from build123d import *

# Parameters (mm, degrees)
EXTRUDE_1_DEPTH     = 2
SKETCH_2_W          = 46
SKETCH_2_H          = 21
EXTRUDE_2_DEPTH     = 5.5
SKETCH_3_R          = 2.5
SKETCH_3_R_2        = 1.5
EXTRUDE_3_DEPTH     = 5.5
CUT_EXTRUDE_2_REACH = 27
SKETCH_5_W          = 12.7
SKETCH_5_H          = 3
EXTRUDE_4_DEPTH     = 7.5
SKETCH_7_R          = 1.5
CUT_EXTRUDE_3_DEPTH = 3
EXTRUDE_5_DEPTH     = 18
EXTRUDE_6_DEPTH     = 18
SKETCH_10_W         = 5
SKETCH_10_H         = 7.5
SKETCH_10_R         = 1.5
EXTRUDE_7_DEPTH     = 5


with BuildPart() as part:
    # 草图1 → 凸台-拉伸1 (new body)
    with BuildSketch(Plane(origin=(0, 0, 0), x_dir=(1, 0, 0), z_dir=(0, 1, 0))):
        with BuildLine():
            Line((-23, 12.5), (23, 12.5))
            ThreePointArc((23, 12.5), (24.414213562, 11.914213562), (25, 10.5))
            Line((25, 10.5), (25, -10.5))
            ThreePointArc((25, -10.5), (24.414213562, -11.914213562), (23, -12.5))
            Line((23, -12.5), (-23, -12.5))
            ThreePointArc((-23, -12.5), (-24.414213562, -11.914213562), (-25, -10.5))
            Line((-25, -10.5), (-25, 10.5))
            ThreePointArc((-25, 10.5), (-24.414213562, 11.914213562), (-23, 12.5))
        make_face()
    extrude(amount=EXTRUDE_1_DEPTH)

    # 草图2 → 凸台-拉伸2 (add)
    with BuildSketch(Plane(origin=(0, 2, 0), x_dir=(1, 0, 0), z_dir=(0, 1, 0))):
        with BuildLine():
            Line((-25, 10.5), (-25, -10.5))
            ThreePointArc((-25, -10.5), (-24.414213562, -11.914213562), (-23, -12.5))
            Line((-23, -12.5), (23, -12.5))
            ThreePointArc((23, -12.5), (24.414213562, -11.914213562), (25, -10.5))
            Line((25, -10.5), (25, 10.5))
            ThreePointArc((25, 10.5), (24.414213562, 11.914213562), (23, 12.5))
            Line((23, 12.5), (-23, 12.5))
            ThreePointArc((-23, 12.5), (-24.414213562, 11.914213562), (-25, 10.5))
        make_face()
        Rectangle(SKETCH_2_W, SKETCH_2_H, mode=Mode.SUBTRACT)
    extrude(amount=EXTRUDE_2_DEPTH)

    # 草图3 → 凸台-拉伸3 (add)
    with BuildSketch(Plane(origin=(0, 2, 0), x_dir=(1, 0, 0), z_dir=(0, 1, 0))):
        with Locations((-21, 8.5)):
            Circle(SKETCH_3_R)
        with Locations((-21, 8.5)):
            Circle(SKETCH_3_R_2, mode=Mode.SUBTRACT)
        with Locations((21, 8.5)):
            Circle(SKETCH_3_R)
        with Locations((21, 8.5)):
            Circle(SKETCH_3_R_2, mode=Mode.SUBTRACT)
        with Locations((21, -8.5)):
            Circle(SKETCH_3_R)
        with Locations((21, -8.5)):
            Circle(SKETCH_3_R_2, mode=Mode.SUBTRACT)
        with Locations((-21, -8.5)):
            Circle(SKETCH_3_R)
        with Locations((-21, -8.5)):
            Circle(SKETCH_3_R_2, mode=Mode.SUBTRACT)
    extrude(amount=EXTRUDE_3_DEPTH)

    # 草图5 → 切除-拉伸2 (cut, up to next)
    with BuildSketch(Plane.XY.offset(12.5), mode=Mode.PRIVATE) as cut_extrude_2_sk1:
        with Locations((0, 3.5)):
            Rectangle(SKETCH_5_W, SKETCH_5_H)
    cut_extrude_2_tool1 = extrude(cut_extrude_2_sk1.sketch, amount=-CUT_EXTRUDE_2_REACH, mode=Mode.PRIVATE) & part.part
    add(cut_extrude_2_tool1.solids().sort_by_distance((0, 3.5, 12.5))[0], mode=Mode.SUBTRACT)

    # 草图6 → 凸台-拉伸4 (add)
    with BuildSketch(Plane.XZ):
        Polygon((23, 12.5), (30, 12.5), (30, 10.5), (25, 10.5), align=None)
        Polygon((-23, 12.5), (-30, 12.5), (-30, 10.5), (-25, 10.5), align=None)
    extrude(amount=-EXTRUDE_4_DEPTH)

    # 草图7 → 切除-拉伸3 (cut, through all)
    with BuildSketch(Plane(origin=(0, 0, 10.5), x_dir=(-1, 0, 0), z_dir=(0, 0, -1))):
        with Locations((-27.5, 3.75)):
            Circle(SKETCH_7_R)
        with Locations((27.5, 3.75)):
            Circle(SKETCH_7_R)
    extrude(amount=-CUT_EXTRUDE_3_DEPTH, mode=Mode.SUBTRACT)

    # 草图8 → 凸台-拉伸5 (add)
    with BuildSketch(Plane.XY.offset(12.5)):
        with BuildLine():
            Line((-29, 7.5), (-29, 3.75))
            ThreePointArc((-29, 3.75), (-27.5, 2.25), (-26, 3.75))
            Line((-26, 3.75), (-26, 7.5))
            Line((-26, 7.5), (-24, 7.5))
            Line((-24, 7.5), (-24, 0))
            Line((-24, 0), (-30, 0))
            Line((-30, 0), (-30, 7.5))
            Line((-30, 7.5), (-29, 7.5))
        make_face()
        with BuildLine():
            Line((29, 7.5), (29, 3.75))
            ThreePointArc((29, 3.75), (27.5, 2.25), (26, 3.75))
            Line((26, 3.75), (26, 7.5))
            Line((26, 7.5), (24, 7.5))
            Line((24, 7.5), (24, 0))
            Line((24, 0), (30, 0))
            Line((30, 0), (30, 7.5))
            Line((30, 7.5), (29, 7.5))
        make_face()
    extrude(amount=EXTRUDE_5_DEPTH)

    # 草图9 → 凸台-拉伸6 (add)
    with BuildSketch(Plane.XY.offset(12.5)):
        with BuildLine():
            Line((29, 3.75), (29, 7.5))
            Line((29, 7.5), (26, 7.5))
            Line((26, 7.5), (26, 3.75))
            ThreePointArc((26, 3.75), (27.5, 5.25), (29, 3.75))
        make_face()
        with BuildLine():
            Line((-29, 7.5), (-29, 3.75))
            ThreePointArc((-29, 3.75), (-27.5, 5.25), (-26, 3.75))
            Line((-26, 3.75), (-26, 7.5))
            Line((-26, 7.5), (-29, 7.5))
        make_face()
    extrude(amount=EXTRUDE_6_DEPTH)

    # 草图10 → 凸台-拉伸7 (add)
    with BuildSketch(Plane(origin=(0, 0, 10.5), x_dir=(-1, 0, 0), z_dir=(0, 0, -1))):
        with Locations((-27.5, 3.75)):
            Rectangle(SKETCH_10_W, SKETCH_10_H)
        with Locations((-27.5, 3.75)):
            Circle(SKETCH_10_R, mode=Mode.SUBTRACT)
        with Locations((27.5, 3.75)):
            Rectangle(SKETCH_10_W, SKETCH_10_H)
        with Locations((27.5, 3.75)):
            Circle(SKETCH_10_R, mode=Mode.SUBTRACT)
    extrude(amount=EXTRUDE_7_DEPTH)


solid = part.part
Input: part model. Units: mm. Frame: model coordinates. A direction names the side the tool comes from. Coordinates: 2 decimals unless noted, no trailing zeros. Loops run counter-clockwise (first coordinate to the right, second up) from the corner with the lowest first, then second, coordinate; pieces in that order, holes last. Notation, with made-up numbers: (-21.75, 53) - (-13.75, 53) arc R23 cw to (-13.75, 66) - close; hole circle Ø11 at (-37, 33.5). An arc over 180 degrees is marked (long way). Answer in a Markdown table with one row per item. Add a question column.
Item 1: Contact query for flat-ended pins moving along their axis: P1, Ø0.9, axis at x = 21, z = 9, coming from the +Y side; P2, Ø3, axis at y = 3.5, z = 0.5, coming from the +X side; P3, Ø1, axis at x = 11.5, y = 4.5, coming from the +Z side. Output: stop coordinate, or through.
Item 2: Section query D-D on z = 8.5. Return the cut outline in (x, y).
Item 3: Section query A-A on x = -27.5. Return the cut outline in (y, z).
Item 4: Access query for faces 5 (the cylindrical face through (-22.5, 4.71, 8.43)), 6 (the flat face through (28, 2, 5.5)), 7 (the flat face through (0, 5, 12)), 8 (the flat face through (-24, 4, 21)). Directions: +Z, -Z, +X, -X, +Y, -Y. A direction counts if a zero-diameter tool reaches every point of the face in a straight line with its end or side. Return the directions, or none.
Item 5: Section query C-C on z = -1.5. Return the cut outline in (x, y).
Item 6: Line query: line 1 along X through (y, z) = (5, -8.5); line 2 along X through (y, z) = (6.3, 8.5); line 3 along Z through (x, y) = (-21, 5.9). Output: solid intervals per line, ascending. Write a range as [from, to].
Item 7: Section query B-B on y = 3.75. State how many separate pieces and enclosed holes the cut face has, then the cut area to 3 significant figures.
Item 8: Mould query, pull axis X, two halves, no side actions, for faces 1 (the flat face through (25.6, 3.8, 30.5)), 2 (the flat face through (-21, 2, 8)), 3 (the cylindrical face through (-22.5, 4.71, -8.57)), 4 (the flat face through (-25, 4, -3)). Classes: released by +X, released by -X, zero draft, split by the parting line, or undercut.
Recorded:
| question | item | result |
|---|---|---|
| 1 | P1 | y = 2 |
| 1 | P2 | x = 25 |
| 1 | P3 | z = 12.5 |
| 2 | outline | (-30, 0) - (30, 0) - (30, 7.5) - (22.5, 7.5) - (22.5, 2) - (19.5, 2) - (19.5, 7.5) - (18.5, 7.5) - (18.5, 2) - (-18.5, 2) - (-18.5, 7.5) - (-19.5, 7.5) - (-19.5, 2) - (-22.5, 2) - (-22.5, 7.5) - (-30, 7.5) - close; hole circle Ø3 at (-27.5, 3.75); hole circle Ø3 at (27.5, 3.75) |
| 3 | outline | (0, 5.5) - (2.25, 5.5) - (2.25, 30.5) - (0, 30.5) - close; (5.25, 5.5) - (7.5, 5.5) - (7.5, 30.5) - (5.25, 30.5) - close |
| 4 | face 5 | +Y |
| 4 | face 6 | -Z, +X, +Y, -Y |
| 4 | face 7 | +Z |
| 4 | face 8 | +Z, +Y, -Y |
| 5 | outline | (-25, 0) - (25, 0) - (25, 7.5) - (23, 7.5) - (23, 2) - (-23, 2) - (-23, 7.5) - (-25, 7.5) - close |
| 6 | line 1 | [-25, -22.5], [-19.5, -18.5], [18.5, 19.5], [22.5, 25] |
| 6 | line 2 | [-30, -22.5], [-19.5, -18.5], [18.5, 19.5], [22.5, 30] |
| 6 | line 3 | [-12.5, -10], [-7, -6], [6, 7], [10, 12.5] |
| 7 | separate pieces | 3 |
| 7 | enclosed holes | 8 |
| 7 | area | 435 mm^2 |
| 8 | face 1 | zero draft |
| 8 | face 2 | undercut |
| 8 | face 3 | undercut |
| 8 | face 4 | released by -X |
